Autodesk Inventor part; units mm, degrees
ref_plane "YZ Plane" through (0, 0, 0) normal (1, 0, 0) x (0, 1, 0)
ref_plane "XZ Plane" through (0, 0, 0) normal (0, 1, 0) x (-1, 0, 0)
ref_plane "XY Plane" through (0, 0, 0) normal (0, 0, 1) x (1, 0, 0)
sketch "Sketch1" plane through (0, 0, 0) normal (0, 1, 0) x (-1, 0, 0)
  line L0 (0, 0) -> (25.4, 0)
  line L1 (25.4, 0) -> (25.4, -25.4)
  line L2 (25.4, -25.4) -> (0, -25.4)
  line L3 (0, -25.4) -> (0, 0)
  line L4 (23.8125, -23.8125) -> (23.8125, -1.5875)
  line L5 (23.8125, -1.5875) -> (1.5875, -1.5875)
  line L6 (1.5875, -1.5875) -> (1.5875, -23.8125)
  line L7 (1.5875, -23.8125) -> (23.8125, -23.8125)
  dimension "d0" = 25.4
  dimension "d1" = 25.4
  dimension "d2" = 1.5875
extrude "Extrusion1" add sketch "Sketch1" along normal blind 577.85
sketch "Sketch2" plane through (0, 0, -25.4) normal (0, 0, -1) x (-1, 0, 0)
  circle A0 centre (12.7, 565.15) radius 6.35
  line L0 (0, 577.85) -> (25.4, 577.85)
  point P0 (0, 0)
  dimension "d5" = 12.7
  dimension "d6" = 12.7
extrude "Extrusion2" cut sketch "Sketch2" against normal blind 25.4
sketch "Sketch4" plane through (-25.4, 0, 0) normal (0, 0, 1) x (1, 0, 0)
  circle A0 centre (13.1572, 12.7) radius 6.35
  line L0 (0, 0) -> (0, 577.85)
  line L1 (25.4, 0) -> (0, 0)
  dimension "d14" = 12.7
  dimension "d15" = 13.1572
  dimension "d16" = 12.7
extrude "Extrusion4" cut sketch "Sketch4" against normal blind 25.4
properties part number "AP 6"
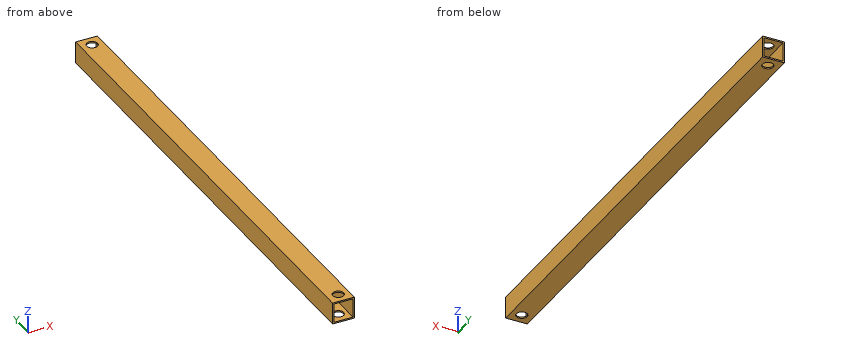
Could you check a few things on this model? Use its own coordinates, in mm. Coordinates: 2 decimals unless noted, no trailing zeros. Write each loop counter-clockwise with the first axis right and the second up, starting at its lowest first coordinate (ties: lowest second). Pieces come first, ordered by that corner, then holes. Notation, with made-up numbers: (5, 14.5) -> (9, 14.5) arc R26 cw to (9, 31.5) -> close; hole circle Ø3 at (17.25, 84.25). An arc over 180 degrees is marked (long way). Write item = value, one per line. Start each with the question number.
(1) I want a section at D-D (x = -12.7). Please give me the cut outline in (y, z), plus the area to 3 significant figures.
(2) I want a section at B-B (z = -13.5). Please give me the cut outline in (x, y), plus the area to 3 significant figures.
(3) I want a section at A-A (y = 565.15). Please give me the cut outline in (x, z), plus the area to 3 significant figures.
(4) Will this pin go through, and if not, where does the flat tip stop? pin 1 (6 mm diameter, centred on x = -19.5, z = -9, fed in from -Y).
(5) I want a section at C-C (y = 327.5). Please give me the cut outline in (x, z).
(6) I need wall thicknesses on line 1 (Y direction, x = -12.7, z = -24.45); line 2 (X direction, y = 565.15, z = -24.15); line 3 (Z direction, x = -16.75, y = 360). Which ranges of each line are inside material? Lowest first, please. Write a range as [from, to].
Result set:
q1.outline = (0, -25.4) -> (6.37, -25.4) -> (6.37, -23.81) -> (0, -23.81) -> close; (0, -1.59) -> (6.37, -1.59) -> (6.37, 0) -> (0, 0) -> close; (19.03, -25.4) -> (558.8, -25.4) -> (558.8, -23.81) -> (19.03, -23.81) -> close; (19.03, -1.59) -> (558.8, -1.59) -> (558.8, 0) -> (19.03, 0) -> close; (571.5, -25.4) -> (577.85, -25.4) -> (577.85, -23.81) -> (571.5, -23.81) -> close; (571.5, -1.59) -> (577.85, -1.59) -> (577.85, 0) -> (571.5, 0) -> close
q1.area = 1,750 mm2
q2.outline = (-25.4, 0) -> (-23.81, 0) -> (-23.81, 577.85) -> (-25.4, 577.85) -> close; (-1.59, 0) -> (0, 0) -> (0, 577.85) -> (-1.59, 577.85) -> close
q2.area = 1,830 mm2
q3.outline = (-25.4, -25.4) -> (-19.05, -25.4) -> (-19.05, -23.81) -> (-23.81, -23.81) -> (-23.81, -1.59) -> (-19.05, -1.59) -> (-19.05, 0) -> (-25.4, 0) -> close; (-6.35, -25.4) -> (0, -25.4) -> (0, 0) -> (-6.35, 0) -> (-6.35, -1.59) -> (-1.59, -1.59) -> (-1.59, -23.81) -> (-6.35, -23.81) -> close
q3.area = 111 mm2
q4.pin_1 = through
q5.outline = (-25.4, -25.4) -> (0, -25.4) -> (0, 0) -> (-25.4, 0) -> close; hole (-23.81, -23.81) -> (-1.59, -23.81) -> (-1.59, -1.59) -> (-23.81, -1.59) -> close
q6.line_1 = [0, 6.37], [19.03, 558.8], [571.5, 577.85]
q6.line_2 = [-25.4, -19.05], [-6.35, 0]
q6.line_3 = [-25.4, -23.81], [-1.59, 0]
